The drawing under review shows one solid part. Ordinate dimensions are in mm from its lowest x, y, z. Round coordinates to 2 decimals unless told otherwise and drop trailing zeros. Write each loop counter-clockwise with the first axis right and the second up, starting at its lowest first coordinate (ties: lowest second). Pieces come first, ordered by that corner, then holes. Notation, with made-up numbers: (33, 24.5) -> (73, 24.5) arc R19 cw to (73, 36.5) -> close; hole circle Ø11 at (-18, 36.5). An arc over 180 degrees is marked (long way). Answer in a Markdown table with one row per item. Add a question column.
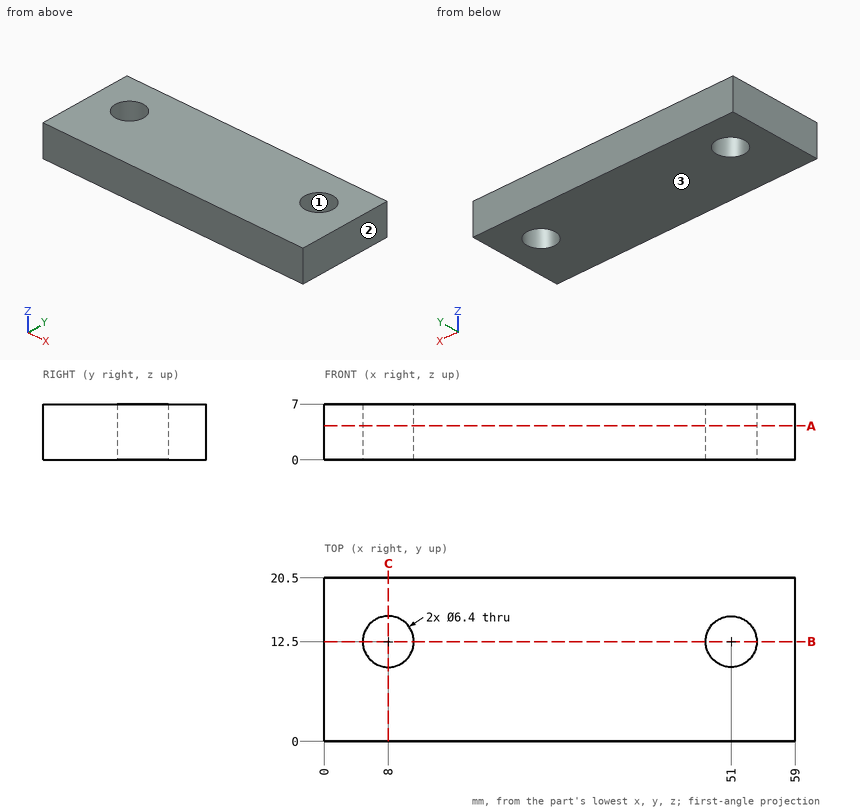
1. Add section A-A on z = 4.25. Write out the cut boundary in (x, y), plus the area to 3 significant figures.
2. Mouldability with a two-part tool opening along X and no side actions: class the marked faces 1, 2 and 3 as pulls with the +X half, pulls with the -X half, needs draft (parallel to the pull), parting line crosses it, or undercut.
3. Add section B-B on y = 12.5. Write out the cut boundary in (x, z), plus the area to 3 significant figures.
4. Add section C-C on x = 8. Write out the cut boundary in (y, z).
5. For L1, parallel to Y at x = 51, z = 4.5; L2, parallel to X at y = 13, z = 2.25; L3, parallel to X at y = 9.75, z = 5.75, list the stretches that pass through material, from the lowest coordinate up.
Filled in:
| question | item | result |
|---|---|---|
| 1 | outline | (0, 0) -> (59, 0) -> (59, 20.5) -> (0, 20.5) -> close; hole circle Ø6.4 at (8, 12.5); hole circle Ø6.4 at (51, 12.5) |
| 1 | area | 1,150 mm² |
| 2 | face 1 | undercut |
| 2 | face 2 | pulls with the +X half |
| 2 | face 3 | needs draft |
| 3 | outline | (0, 0) -> (4.8, 0) -> (4.8, 7) -> (0, 7) -> close; (11.2, 0) -> (47.8, 0) -> (47.8, 7) -> (11.2, 7) -> close; (54.2, 0) -> (59, 0) -> (59, 7) -> (54.2, 7) -> close |
| 3 | area | 323 mm² |
| 4 | outline | (0, 0) -> (9.3, 0) -> (9.3, 7) -> (0, 7) -> close; (15.7, 0) -> (20.5, 0) -> (20.5, 7) -> (15.7, 7) -> close |
| 5 | L1 | 0 to 9.3, 15.7 to 20.5 |
| 5 | L2 | 0 to 4.84, 11.16 to 47.84, 54.16 to 59 |
| 5 | L3 | 0 to 6.36, 9.64 to 49.36, 52.64 to 59 |
